```python
from build123d import *

# Parameters (mm, degrees)
F0_R     = 11
F0_R_2   = 8
F1_DEPTH = 8.33
F2_R     = 11.5325347533
F2_R_2   = 11
F3_DEPTH = 25


# Not quite as in the source:
# - a fillet or chamfer that OpenCascade refuses, or shapes differently, is made with other operations: its cross-section is extruded or revolved along the edge and cut away or added


with BuildPart() as f1:
    # F0 (on Top) → F1 (new body)
    with BuildSketch(Plane.XY):
        Circle(F0_R)
        Circle(F0_R_2, mode=Mode.SUBTRACT)
    extrude(amount=F1_DEPTH)

    # F2 (on face) → F3 (cut)
    with BuildSketch(Plane.XY.offset(8.33)):
        Circle(F2_R)
        Circle(F2_R_2, mode=Mode.SUBTRACT)
    extrude(amount=-F3_DEPTH, mode=Mode.SUBTRACT)

    # F4: fillet of radius 5 on 1 edges, made by hand

    # F4_s1 → F4_t2 (revolve, cut)
    with BuildSketch(Plane.XZ):
        with BuildLine():
            ThreePointArc((8, 3.747424305), (8.8166998673, 6.4860370926), (11, 8.33))
            Line((11, 8.33), (8, 8.33))
            Line((8, 8.33), (8, 3.747424305))
        make_face()
    revolve(axis=Axis((0, 0, 8.33), (0, 0, 1)), mode=Mode.SUBTRACT)

    # F5: fillet of radius 4 on 1 edges, made by hand

    # F5_s1 → F5_t2 (revolve, cut)
    with BuildSketch(Plane.XZ):
        with BuildLine():
            ThreePointArc((11, 0), (8.6975924738, 1.6252394507), (8.0383219615, 4.3652843555))
            Line((8.0383219615, 4.3652843555), (7.6413877184, 4.4147131595))
            ThreePointArc((7.6413877184, 4.4147131595), (7.6, 3.747424305), (7.6, 0))
            Line((7.6, 0), (8, -0.4))
            ThreePointArc((8, -0.4), (9.5, -0.4), (10.8992335608, -0.3870996315))
            Line((10.8992335608, -0.3870996315), (11, 0))
        make_face()
    revolve(axis=Axis((0, 0, 0), (0, 0, 1)), mode=Mode.SUBTRACT)


solid = f1.part
```
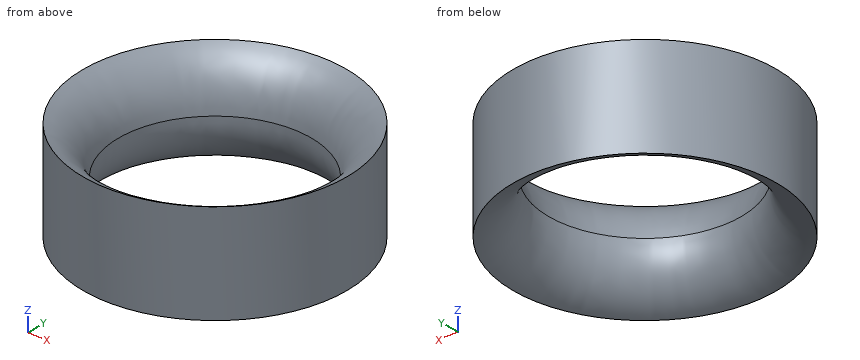
Input: part model. Units: mm. Frame: model coordinates. Give positions to 0.01 mm unless a question says otherwise; leave off trailing zeros. Order: outer loops, then holes, each group sorted by start corner. A loop starts at its lowest first (then second) coordinate and runs counter-clockwise, first axis right, second up. Notation, with made-up numbers: (-0.75, 34) -> (48.25, 34) arc R14 cw to (48.25, 39) -> close; hole circle Ø11 at (-6.5, 47.25). An arc over 180 degrees is marked (long way). Write each question's results on one line, items separated by ' | '. Start each with the question number.
Item 1: Cut plane D-D on z = 1.5. Return the cut outline in (x, y), then the cut area to 3 significant figures.
Item 2: Cut plane A-A on y = 0. Return the cut outline in (x, z).
Item 3: Line query: line 1 (Y direction, x = 3.75, z = 1.5); line 2 (Y direction, x = 4.75, z = 0.5); line 3 (X direction, y = 4.25, z = 4). Output: solid intervals per line, ascending.
Item 4: Contact query for flat-ended pins moving along their axis: P1, Ø5, axis at x = -7, y = 3, coming from the +Z side; P2, Ø3, axis at y = 7.5, z = 2, coming from the +X side; P3, Ø2, axis at x = 6.5, y = -6, coming from the +Z side. Output: stop coordinate, or through.
Item 5: Cut plane C-C on z = 6.5. Return the cut outline in (x, y), then the cut area to 3 significant figures.
Established:
1) outline: circle Ø22 at (0, 0); hole circle Ø17.57 at (0, 0) | area: 138 mm^2
2) outline: (-11, 0) arc R4 ccw to (-8.04, 4.37) arc R5 ccw to (-11, 8.33) -> close; (8.04, 4.37) arc R4 ccw to (11, 0) -> (11, 8.33) arc R5 ccw to start
3) line 1: -10.34 to -7.95, 7.95 to 10.34 | line 2: -9.92 to -8.63, 8.63 to 9.92 | line 3: -10.15 to -6.79, 6.79 to 10.15
4) P1: z = 7.83 | P2: x = 9.22 | P3: z = 7.63
5) outline: circle Ø22 at (0, 0); hole circle Ø17.65 at (0, 0) | area: 135 mm^2
